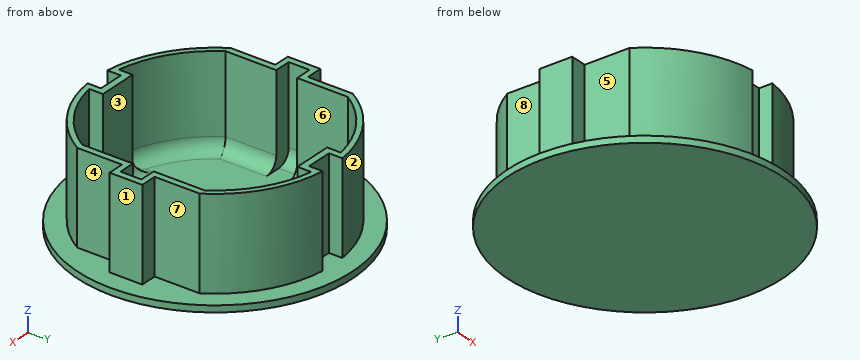
from build123d import *

# Parameters (mm, degrees)
F0_R     = 21
F1_DEPTH = 1
F2_DEPTH = 15
F4_DEPTH = 14
F5_R     = 2


with BuildPart() as f1:
    # F0 (on Top) → F1 (new body)
    with BuildSketch(Plane.XY):
        Circle(F0_R)
        with BuildLine():
            Line((-15.5, -2.5), (-18, -2.5))
            Line((-18, -2.5), (-18, 0))
            Line((-18, 0), (-18, 2.5))
            Line((-18, 2.5), (-15.5, 2.5))
            Line((-15.5, 2.5), (-15.5, 9.367497))
            ThreePointArc((-15.5, 9.367497), (-9.756666, 15.25803), (-2, 18))
            Line((-2, 18), (-2, 15.938399))
            Line((-2, 15.938399), (0, 15.938399))
            Line((0, 15.938399), (2, 15.938399))
            Line((2, 15.938399), (2, 18))
            ThreePointArc((2, 18), (9.756666, 15.25803), (15.5, 9.367497))
            Line((15.5, 9.367497), (15.5, 2.5))
            Line((15.5, 2.5), (18, 2.5))
            Line((18, 2.5), (18, 0))
            Line((18, 0), (18, -2.5))
            Line((18, -2.5), (15.5, -2.5))
            Line((15.5, -2.5), (15.5, -9.367497))
            ThreePointArc((15.5, -9.367497), (9.756666, -15.25803), (2, -18))
            Line((2, -18), (2, -15.938399))
            Line((2, -15.938399), (0, -15.938399))
            Line((0, -15.938399), (-2, -15.938399))
            Line((-2, -15.938399), (-2, -18))
            ThreePointArc((-2, -18), (-9.756666, -15.25803), (-15.5, -9.367497))
            Line((-15.5, -9.367497), (-15.5, -2.5))
        make_face(mode=Mode.SUBTRACT)
        with BuildLine():
            Line((-18, 0), (-18, -2.5))
            Line((-18, -2.5), (-15.5, -2.5))
            Line((-15.5, -2.5), (-15.5, -9.367497))
            ThreePointArc((-15.5, -9.367497), (-9.756666, -15.25803), (-2, -18))
            Line((-2, -18), (-2, -15.938399))
            Line((-2, -15.938399), (0, -15.938399))
            Line((0, -15.938399), (2, -15.938399))
            Line((2, -15.938399), (2, -18))
            ThreePointArc((2, -18), (9.756666, -15.25803), (15.5, -9.367497))
            Line((15.5, -9.367497), (15.5, -2.5))
            Line((15.5, -2.5), (18, -2.5))
            Line((18, -2.5), (18, 0))
            Line((18, 0), (18, 2.5))
            Line((18, 2.5), (15.5, 2.5))
            Line((15.5, 2.5), (15.5, 9.367497))
            ThreePointArc((15.5, 9.367497), (9.756666, 15.25803), (2, 18))
            Line((2, 18), (2, 15.938399))
            Line((2, 15.938399), (0, 15.938399))
            Line((0, 15.938399), (-2, 15.938399))
            Line((-2, 15.938399), (-2, 18))
            ThreePointArc((-2, 18), (-9.756666, 15.25803), (-15.5, 9.367497))
            Line((-15.5, 9.367497), (-15.5, 2.5))
            Line((-15.5, 2.5), (-18, 2.5))
            Line((-18, 2.5), (-18, 0))
        make_face()
    extrude(amount=F1_DEPTH)

    # F0 (on Top) → F2 (join)
    with BuildSketch(Plane.XY):
        with BuildLine():
            Line((-18, 0), (-18, -2.5))
            Line((-18, -2.5), (-15.5, -2.5))
            Line((-15.5, -2.5), (-15.5, -9.367497))
            ThreePointArc((-15.5, -9.367497), (-9.756666, -15.25803), (-2, -18))
            Line((-2, -18), (-2, -15.938399))
            Line((-2, -15.938399), (0, -15.938399))
            Line((0, -15.938399), (2, -15.938399))
            Line((2, -15.938399), (2, -18))
            ThreePointArc((2, -18), (9.756666, -15.25803), (15.5, -9.367497))
            Line((15.5, -9.367497), (15.5, -2.5))
            Line((15.5, -2.5), (18, -2.5))
            Line((18, -2.5), (18, 0))
            Line((18, 0), (18, 2.5))
            Line((18, 2.5), (15.5, 2.5))
            Line((15.5, 2.5), (15.5, 9.367497))
            ThreePointArc((15.5, 9.367497), (9.756666, 15.25803), (2, 18))
            Line((2, 18), (2, 15.938399))
            Line((2, 15.938399), (0, 15.938399))
            Line((0, 15.938399), (-2, 15.938399))
            Line((-2, 15.938399), (-2, 18))
            ThreePointArc((-2, 18), (-9.756666, 15.25803), (-15.5, 9.367497))
            Line((-15.5, 9.367497), (-15.5, 2.5))
            Line((-15.5, 2.5), (-18, 2.5))
            Line((-18, 2.5), (-18, 0))
        make_face()
    extrude(amount=F2_DEPTH)

    # F3 (on face) → F4 (cut)
    with BuildSketch(Plane.XY.offset(15)):
        with BuildLine():
            Line((-17, 0), (-17, -1.6))
            Line((-17, -1.6), (-14.5, -1.6))
            Line((-14.5, -1.6), (-14.5, -9.367497))
            ThreePointArc((-14.5, -9.367497), (-9.546008, -14.383106), (-3, -17))
            Line((-3, -17), (-3, -14.9))
            Line((-3, -14.9), (0, -14.9))
            Line((0, -14.9), (3, -14.9))
            Line((3, -14.9), (3, -17))
            ThreePointArc((3, -17), (9.546008, -14.383106), (14.5, -9.367497))
            Line((14.5, -9.367497), (14.5, -1.6))
            Line((14.5, -1.6), (17, -1.6))
            Line((17, -1.6), (17, 0))
            Line((17, 0), (17, 1.6))
            Line((17, 1.6), (14.5, 1.6))
            Line((14.5, 1.6), (14.5, 9.367497))
            ThreePointArc((14.5, 9.367497), (9.546008, 14.383106), (3, 17))
            Line((3, 17), (3, 14.9))
            Line((3, 14.9), (0, 14.9))
            Line((0, 14.9), (-3, 14.9))
            Line((-3, 14.9), (-3, 17))
            ThreePointArc((-3, 17), (-9.546008, 14.383106), (-14.5, 9.367497))
            Line((-14.5, 9.367497), (-14.5, 1.6))
            Line((-14.5, 1.6), (-17, 1.6))
            Line((-17, 1.6), (-17, 0))
        make_face()
    extrude(amount=-F4_DEPTH, mode=Mode.SUBTRACT)

    # F5
    f5_edges = [f1.edges().sort_by_distance(p)[0] for p in [
        (-14.5, -5.483748, 1),
        (-17, 0, 1),
        (-14.5, 5.483748, 1),
        (-9.546008, 14.383106, 1),
        (-9.546008, -14.383106, 1),
        (9.546008, -14.383106, 1),
        (0, -14.9, 1),
        (14.5, -5.483748, 1),
        (14.5, 5.483748, 1),
        (17, 0, 1),
        (9.546008, 14.383106, 1),
        (0, 14.9, 1),
        (3, -15.95, 1),
        (-3, -15.95, 1),
        (3, 15.95, 1),
        (-3, 15.95, 1),
    ]]
    fillet(f5_edges, radius=F5_R)


solid = f1.part
Verification items for the finished model (mm, model axes). Face numbers are marked on the shaded views. A direction names the side the tool comes from. Coordinates: 2 decimals unless noted, no trailing zeros. Write each loop counter-clockwise with the first axis right and the second up, starting at its lowest first coordinate (ties: lowest second). Pieces come first, ordered by that corner, then holes. Notation, with made-up numbers: (-29.75, 52.25) - (15.25, 52.25) arc R26 ccw to (15.25, 82.25) - close; hole circle Ø5 at (18, -37). An arc over 180 degrees is marked (long way). Answer as a JSON object with one key per item and string values.
(1) Gauge pin test, flat ends, axial feed: pin 1 Ø1 at (y, z) = (16, 8.5) entering from -X; pin 2 Ø6.5 at (x, z) = (0.5, 10.5) entering from +Y; pin 3 Ø0.6 at (y, z) = (-17, 8) entering from -X. Record the tip position at first contact, or that the pin passes through.
Report:
{"pin 1": "x = -9.37", "pin 2": "y = 18", "pin 3": "x = -7.01"}
(2) Cross-section at B-B on x = 0. Record the cut outline in (y, z), plus the area to 3 significant figures.
Report:
{"outline": "(-21, 0) - (21, 0) - (21, 1) - (15.94, 1) - (15.94, 15) - (14.9, 15) - (14.9, 3) arc R2 cw to (12.9, 1) - (-12.9, 1) arc R2 cw to (-14.9, 3) - (-14.9, 15) - (-15.94, 15) - (-15.94, 1) - (-21, 1) - close", "area": "72.8 mm^2"}
(3) Cross-section at A-A on y = 0. Record the cut outline in (x, z), plus the area to 3 significant figures.
Report:
{"outline": "(-21, 0) - (21, 0) - (21, 1) - (18, 1) - (18, 15) - (17, 15) - (17, 3) arc R2 cw to (15, 1) - (-15, 1) arc R2 cw to (-17, 3) - (-17, 15) - (-18, 15) - (-18, 1) - (-21, 1) - close", "area": "71.7 mm^2"}
(4) Thickness scan on line 1 along X through (y, z) = (3, 6.5); line 2 along X through (y, z) = (0, 5); line 3 along Z through (x, y) = (-16, 3). Record the ranges inside material, lowest first.
Report:
{"line 1": "-15.5 to -14.5, 14.5 to 15.5", "line 2": "-18 to -17, 17 to 18", "line 3": "0 to 1"}
(5) Tool access check on the marked faces 1, 2, 3, 4 and 5. Record the directions out of +Z, -Z, +X, -X, +Y, -Y that give a thin tool (end or side, any length) a straight path to the whole face; none if there is none.
Report:
{"face 1": "+Z, +X, +Y, -Y", "face 2": "+Z, -X, +Y", "face 3": "+Z", "face 4": "+Z, +X, -Y", "face 5": "+Z, -X, -Y"}
(6) Mould release check, pull along X, two halves, no side actions. Record for the marked faces 6, 7 and 8: pulls with the +X half, pulls with the -X half, needs draft (parallel to the pull), parting line crosses it, or undercut.
Report:
{"face 6": "undercut", "face 7": "pulls with the +X half", "face 8": "pulls with the -X half"}
